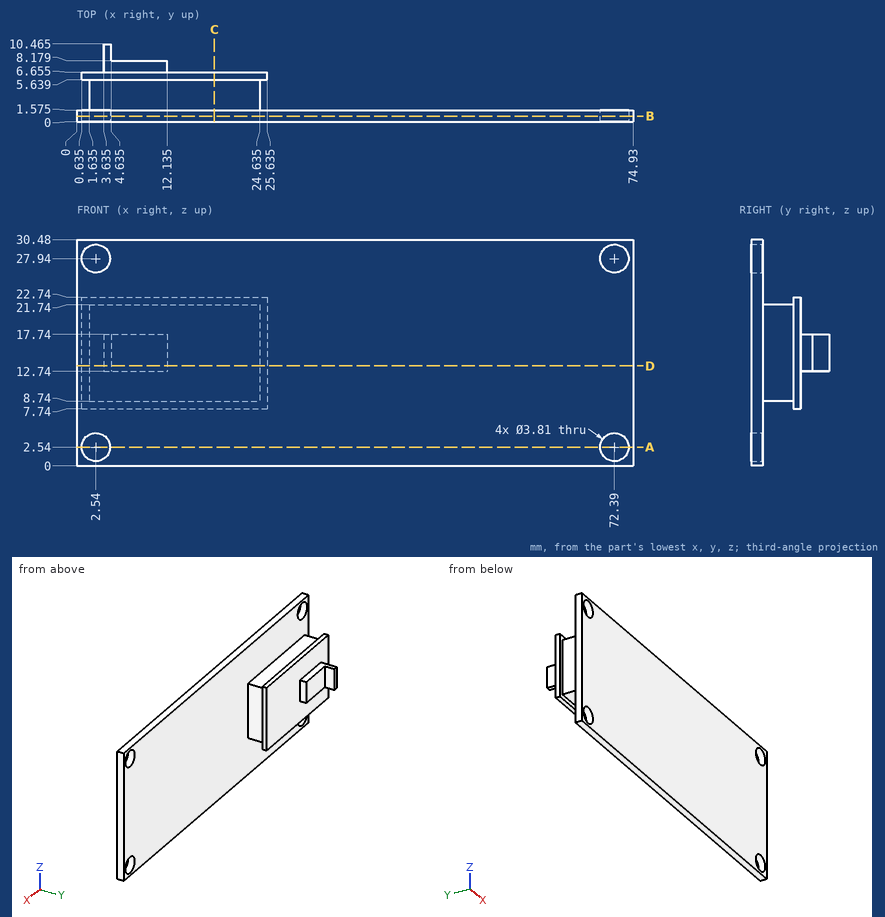
The drawing under review shows one solid part. Ordinate dimensions are in mm from its lowest x, y, z. Round coordinates to 2 decimals unless told otherwise and drop trailing zeros. Loops run counter-clockwise (first coordinate to the right, second up) from the corner with the lowest first, then second, coordinate; pieces in that order, holes last. Notation, with made-up numbers: (88.25, -29.5) - (110.25, -29.5) arc R28 cw to (110.25, -5.5) - close; hole circle Ø3 at (89, -17.5). An arc over 180 degrees is marked (long way). One line per question, with ' | ' between items.
Q1. Take a section at D-D (z = 13.5). Give the boundary of the cut face in (x, y) (1 decimal).
Taken from the geometry:
outline: (0, 0) - (74.9, 0) - (74.9, 1.6) - (24.6, 1.6) - (24.6, 5.6) - (25.6, 5.6) - (25.6, 6.7) - (12.1, 6.7) - (12.1, 8.2) - (4.6, 8.2) - (4.6, 10.5) - (3.6, 10.5) - (3.6, 6.7) - (0.6, 6.7) - (0.6, 5.6) - (1.6, 5.6) - (1.6, 1.6) - (0, 1.6) - close
Q2. For line 1 along Z through (x, y) = (72.39, 1.2) (3 decimals); line 2 along X through (y, z) = (0.6, 27.94) (3 decimals); line 3 along Z through (x, y) = (19, 3.25), list the stretches that pass through material, from the lowest coordinate up. Write a range as [from, to].
Taken from the geometry:
line 1: z = [0, 0.635], [4.445, 26.035], [29.845, 30.48] | line 2: x = [0, 0.635], [4.445, 70.485], [74.295, 74.93] | line 3: z = [8.74, 21.74]
Q3. For pin 1 (4.5 mm diameter, centred on x = 2.54, z = 27.94, fed in from +Y) (3 decimals); pin 2 (3.5 mm diameter, centred on y = 2.5, z = 18.5, fed in from +X); pin 3 (3 mm diameter, centred on y = 8, z = 18, fed in from -X) (3 decimals); pin 4 (2 mm diameter, centred on x = 7.5, y = 4, fed in from +Z), all flat-tipped, find the tip position at first contact; note any pin that passes through.
Taken from the geometry:
pin 1: stops at y = 1.575 | pin 2: stops at x = 74.93 | pin 3: stops at x = 0.635 | pin 4: stops at z = 21.74
Q4. Take a section at A-A (z = 2.54). Give the boundary of the cut face in (x, y) (1 decimal), and give its area (3 significant figures).
Taken from the geometry:
outline: (0, 0) - (0.6, 0) - (0.6, 1.6) - (0, 1.6) - close; (4.4, 0) - (70.5, 0) - (70.5, 1.6) - (4.4, 1.6) - close; (74.3, 0) - (74.9, 0) - (74.9, 1.6) - (74.3, 1.6) - close | area: 106 mm²
Q5. Take a section at B-B (y = 0.75). Give the boundary of the cut face in (x, z) (3 decimals), and give its area (3 significant figures).
Taken from the geometry:
outline: (0, 0) - (74.93, 0) - (74.93, 30.48) - (0, 30.48) - close; hole circle Ø3.81 at (2.54, 2.54); hole circle Ø3.81 at (2.54, 27.94); hole circle Ø3.81 at (72.39, 2.54); hole circle Ø3.81 at (72.39, 27.94) | area: 2,240 mm²
Q6. Take a section at C-C (x = 18.5). Give the boundary of the cut face in (y, z) (1 decimal).
Taken from the geometry:
outline: (0, 0) - (1.6, 0) - (1.6, 8.7) - (5.6, 8.7) - (5.6, 7.7) - (6.7, 7.7) - (6.7, 22.7) - (5.6, 22.7) - (5.6, 21.7) - (1.6, 21.7) - (1.6, 30.5) - (0, 30.5) - close
